```python
from build123d import *

# Parameters (mm, degrees)
SKETCH1_R           = 1
BOSS_EXTRUDE2_DEPTH = 1.6


with BuildPart() as part:
    # Sketch1 → Boss-Extrude2 (new body)
    with BuildSketch(Plane.XY):
        with BuildLine():
            Line((0, 0), (22, 0))
            ThreePointArc((22, 0), (30.128904766, 5.736453046), (24.39245172, 13.865357811))
            ThreePointArc((24.39245172, 13.865357811), (21.823365484, 12.765579929), (22.861725051, 10.171061692))
            ThreePointArc((22.861725051, 10.171061692), (24.759347978, 6.760381893), (22, 4))
            Line((22, 4), (0, 4))
            ThreePointArc((0, 4), (-5.239174154, 2.513368319), (-8.916737512, -1.503414886))
            ThreePointArc((-8.916737512, -1.503414886), (-8.025548834, -4.187773792), (-5.341189927, -3.296585114))
            ThreePointArc((-5.341189927, -3.296585114), (-3.138303015, -0.890503073), (0, 0))
        make_face()
        with Locations((-7.128963719, -2.4)):
            Circle(SKETCH1_R, mode=Mode.SUBTRACT)
        with Locations((23.671036281, 12)):
            Circle(SKETCH1_R, mode=Mode.SUBTRACT)
    extrude(amount=BOSS_EXTRUDE2_DEPTH)


solid = part.part
```
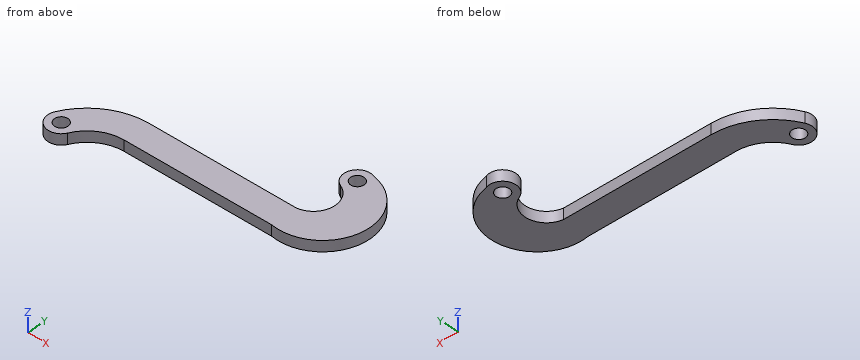
Can you work these out from the model? Positions are in its coordinate system, mm. Round coordinates to 2 decimals unless told otherwise and drop trailing zeros. Order: outer loops, then holes, each group sorted by start corner. A loop starts at its lowest first (then second) coordinate and runs counter-clockwise, first axis right, second up.
(1) I'm going to push flat-ended pins straight in: pin 1 (0.8 mm diameter, centred on x = 7, z = 1, fed in from +Y); pin 2 (1.8 mm diameter, centred on x = -7.13, y = -2.4, fed in from -Z). Where does each tip first touch, or does it pass through?
Results are:
pin 1: stops at y = 4
pin 2: passes through
(2) If I drill on L1, parallel to Y at x = 11.5, z = 1; L2, parallel to Y at x = 26, z = 0.2; L3, parallel to X at y = 7, z = 0.95, over which ranges is the centre line in solid material (lowest first)?
Results are:
L1: y = 0 to 4
L2: y = 0.48 to 13.38
L3: x = 24.78 to 30.23
(3) If we section it at A-A (y = -2.4): Please give me the cut outline in (x, z), plus the area to 3 significant figures.
Results are:
outline: (-9.13, 0) - (-8.13, 0) - (-8.13, 1.6) - (-9.13, 1.6) - close; (-6.13, 0) - (-4.79, 0) - (-4.79, 1.6) - (-6.13, 1.6) - close
area: 3.75 mm2
(4) If we section it at B-B (x = 13): Please give me the cut outline in (y, z).
Results are:
outline: (0, 0) - (4, 0) - (4, 1.6) - (0, 1.6) - close
(5) If we section it at D-D (y = 11.5): Please give me the cut outline in (x, z), plus the area to 3 significant figures.
Results are:
outline: (21.73, 0) - (22.81, 0) - (22.81, 1.6) - (21.73, 1.6) - close; (24.54, 0) - (28.55, 0) - (28.55, 1.6) - (24.54, 1.6) - close
area: 8.13 mm2
